Could you check a few things on this model? Use its own coordinates, in mm. A direction names the side the tool comes from. Round coordinates to 2 decimals unless told otherwise and drop trailing zeros. Loops run counter-clockwise (first coordinate to the right, second up) from the corner with the lowest first, then second, coordinate; pieces in that order, holes last. Notation, with made-up numbers: (-30.5, 36) -> (2.5, 36) arc R11 ccw to (2.5, 47) -> close; hole circle Ø9 at (-24.75, 38). An arc over 180 degrees is marked (long way). One line per item, written item: value.
from build123d import *

# Parameters (mm, degrees)
F1_DEPTH = 36.5125
F2_W     = 54.61
F2_H     = 1.27
F3_DEPTH = 1.5875
F4_SIZE  = 0.79374
F5_W     = 25.4
F5_H     = 38.1
F6_DEPTH = 0.254


# Not quite as in the source:
# - a fillet or chamfer is up to 0.001 mm smaller than in the source, because OpenCascade refuses the exact size


with BuildPart() as f1:
    # F0 (on Front) → F1 (new body, symmetric)
    with BuildSketch(Plane.XZ):
        Polygon((27.305, 0), (30.48, 0), (30.48, 1.5875), (28.8925, 1.5875), (28.8925, 3.96875), (0, 3.96875), (0, 2.8575), (27.305, 2.8575), (27.305, 1.5875), (0, 1.5875), (0, 0), align=None)
        Polygon((-27.305, 0), (0, 0), (0, 1.5875), (-27.305, 1.5875), (-27.305, 2.8575), (0, 2.8575), (0, 3.96875), (-28.8925, 3.96875), (-28.8925, 1.5875), (-30.48, 1.5875), (-30.48, 0), align=None)
    extrude(amount=F1_DEPTH, both=True)

    # F2 (on face) → F3 (join)
    with BuildSketch(Plane(origin=(0, 36.5125, 0), x_dir=(-1, 0, 0), z_dir=(0, 1, 0))):
        Polygon((-30.48, 1.5875), (-30.48, 0), (30.48, 0), (30.48, 1.5875), (28.8925, 1.5875), (28.8925, 3.96875), (-28.8925, 3.96875), (-28.8925, 1.5875), align=None)
        with Locations((0, 2.2225)):
            Rectangle(F2_W, F2_H, mode=Mode.SUBTRACT)
        with Locations((0, 2.2225)):
            Rectangle(F2_W, F2_H)
    extrude(amount=F3_DEPTH)

    # F4 (size 0.79375 in the source; OpenCascade refuses exactly that, so slightly less here)
    f4_edges = [f1.edges().sort_by_distance(p)[0] for p in [
        (27.305, -36.5125, 2.2225),
        (0, -36.5125, 1.5875),
        (0, -36.5125, 2.8575),
        (-27.305, -36.5125, 2.2225),
        (29.68625, 38.1, 1.5875),
        (28.8925, 38.1, 2.778125),
        (0, 38.1, 3.96875),
        (0, 38.1, 0),
        (30.48, 38.1, 0.79375),
        (-28.8925, 38.1, 2.778125),
        (-29.68625, 38.1, 1.5875),
        (-30.48, 38.1, 0.79375),
    ]]
    chamfer(f4_edges, length=F4_SIZE)

    # F5 (on face) → F6 (cut)
    with BuildSketch(Plane(origin=(0, 0, 0), x_dir=(1, 0, 0), z_dir=(0, 0, -1))):
        Rectangle(F5_W, F5_H)
    extrude(amount=-F6_DEPTH, mode=Mode.SUBTRACT)


solid = f1.part
(1) Thinking about a two-plate mould opening in X: for faces 1 (the face through (-30, 0, 1.588)), 2 (the face through (-30.48, 0, 1)), 3 (the face through (0, 0, 0.254)), which applies, released by +X, released by -X, zero draft, split by the parting line, or undercut?
Recorded:
face 1: zero draft
face 2: released by -X
face 3: undercut
(2) I'm going to push flat-ended pins straight in: pin 1 Ø0.8 at (x, y) = (30, -16) entering from +Z; pin 2 Ø0.6 at (y, z) = (-14, 2) entering from +X; pin 3 Ø6 at (x, y) = (4, -2.5) entering from -Z. Where does each tip first touch, or does it pass through?
Recorded:
pin 1: z = 1.59
pin 2: x = 28.89
pin 3: z = 0.25
(3) For faces 4 (the face through (-28.892, 0, 3)), 5 (the face through (0, 0, 1.588)), 6 (the face through (30, 0, 1.588)), 7 (the face through (0, 38.1, 2)), 8 (the face through (-0.1, -36.512, 0.2)), which set-ups out of +Z, -Z, +X, -X, +Y, -Y let a thin tool reach every point of the face, with its end or its side?
Recorded:
face 4: +Z, -X, +Y, -Y
face 5: -Y
face 6: +Z, +X, +Y, -Y
face 7: +Z, -Z, +X, -X, +Y
face 8: +Z, -Z, +X, -X, -Y
(4) If we section it at A-A, the plane y = 29: Please give me the cut outline in (x, z) (1 decimal).
Recorded:
outline: (-30.5, 0) -> (30.5, 0) -> (30.5, 1.6) -> (28.9, 1.6) -> (28.9, 4) -> (-28.9, 4) -> (-28.9, 1.6) -> (-30.5, 1.6) -> close; hole (-27.3, 1.6) -> (27.3, 1.6) -> (27.3, 2.9) -> (-27.3, 2.9) -> close
(5) If I drill on L1, parallel to Z at x = -5.5, y = 16; L2, parallel to Z at x = 19, y = 22; L3, parallel to X at y = 31.5, z = 1.95 (1 decimal), over which ranges is the centre line in solid material (lowest first)?
Recorded:
L1: 0.25 to 1.59, 2.86 to 3.97
L2: 0 to 1.59, 2.86 to 3.97
L3: -28.9 to -27.3, 27.3 to 28.9
